Read the model definition and answer for the solid it produces. Units are mm, in the model's axes. A direction names the side the tool comes from. Coordinates: 2 decimals unless noted, no trailing zeros. Order: outer loops, then holes, each group sorted by start corner. A loop starts at its lowest first (then second) coordinate and runs counter-clockwise, first axis right, second up. Notation, with made-up numbers: (85, -10.5) -> (130, -10.5) arc R13 ccw to (130, 10.5) -> close; hole circle Ø1 at (22, 6). An arc over 180 degrees is marked (long way). Use CSV: the item, a comma, the result in double quotes.
```python
from build123d import *

# Parameters (mm, degrees)
BOSS_EXTRUDE1_DEPTH = 50
FILLET1_R           = 4
CUT_EXTRUDE1_DEPTH  = 1.5


with BuildPart() as part:
    # Sketch1 → Boss-Extrude1 (new body)
    with BuildSketch(Plane.XY):
        Polygon((0, 0), (15, 32.788635103), (15, 40), (-3.299023369, 0), align=None)
    extrude(amount=BOSS_EXTRUDE1_DEPTH)

    # Fillet1
    fillet1_edges = [part.edges().sort_by_distance(p)[0] for p in [
        (-1.649511685, 0, 50),
        (-1.649511685, 0, 0),
    ]]
    fillet(fillet1_edges, radius=FILLET1_R)

    # Sketch2 → Cut-Extrude1 (cut)
    with BuildSketch(Plane(origin=(-2.728080099, 1.248030037, 0), x_dir=(0, 0, 1), z_dir=(-0.9093600329934255, 0.4160100123725345, 0))):
        Polygon((20, 12.820411289), (30, 12.820411289), (34.5, 16.820411289), (34.5, 26.820411289), (36.5, 26.820411289), (36.5, 32.820411289), (26, 32.820411289), (26, 26.820411289), (28, 26.820411289), (28, 18.820411289), (22, 18.820411289), (22, 26.820411289), (24, 26.820411289), (24, 32.820411289), (13.5, 32.820411289), (13.5, 26.820411289), (15.5, 26.820411289), (15.5, 16.820411289), align=None)
    extrude(amount=-CUT_EXTRUDE1_DEPTH, mode=Mode.SUBTRACT)


solid = part.part
```
Item 1: A tool of negligible diameter and unlimited length cuts with its end or side. For faces 1 (the flat face through (7, 22, 22)), 2 (the flat face through (3.278, 12.599, 24.93)), 3 (the flat face through (5.774, 18.055, 25.042)), from which of +Z, -Z, +X, -X, +Y, -Y can it reach the whole face along a straight path? Write none if from no direction.
Return value:
face 1,"-X, +Y"
face 2,"+Y"
face 3,"-X"
Item 2: Each of these flat-tipped pins is pushed along its axis until it touches: P1, Ø2, axis at x = 9, z = 21.5, coming from the +Y side; P2, Ø2, axis at y = 30, z = 34, coming from the +X side; P3, Ø3, axis at y = 20, z = 25.5, coming from the +X side; P4, Ø1.9, axis at x = 10, y = 29.5, coming from the -Z side. Where does it stop, or does it pass through?
Return value:
P1,"stops at y = 25.64"
P2,"stops at x = 14.18"
P3,"stops at x = 9.84"
P4,"stops at z = 0"
Item 3: Find section D-D, the plane y = 14. Give the vertices of the cut face in (x, z).
Return value:
outline,"(3.11, 0) -> (6.4, 0) -> (6.4, 50) -> (3.11, 50) -> (3.11, 31.35) -> (4.76, 32.12) -> (4.76, 17.88) -> (3.11, 18.65) -> close"
Item 4: The mould has two halves that part along X. Classify faces 4 (the flat face through (15, 36, 25)), 5 (the cylindrical face through (-0.699, 1.141, 48.797)), 6 (the flat face through (5.98, 20.28, 24.65)), 7 (the flat face through (4.12, 14.44, 17.72)): +X half, -X half, draft (parallel to the pull), parting line (faces both ways), or undercut.
Return value:
face 4,"+X half"
face 5,"draft"
face 6,"-X half"
face 7,"undercut"
Item 5: Straight lines are drawn through the part: line 1 along Y through (x, z) = (11, 17.5) (3 decimals); line 2 along X through (y, z) = (4, 37.5); line 3 along X through (y, z) = (8, 30.5). For each, find the intervals that lie inside material, in ascending order.
Return value:
line 1,"y = 24.045 to 27.651, 31.06 to 31.256"
line 2,"x = -1.47 to 1.83"
line 3,"x = 0.36 to 3.66"
Item 6: Find section C-C, the plane x = 9. Give the vertices of the cut face in (y, z), then the cut area to 3 significant figures.
Return value:
outline,"(19.67, 0) -> (26.88, 0) -> (26.88, 13.5) -> (25.38, 13.5) -> (25.38, 15.5) -> (23.28, 15.5) -> (23.28, 22) -> (25.38, 22) -> (25.38, 24) -> (26.88, 24) -> (26.88, 26) -> (25.38, 26) -> (25.38, 28) -> (23.28, 28) -> (23.28, 34.5) -> (25.38, 34.5) -> (25.38, 36.5) -> (26.88, 36.5) -> (26.88, 50) -> (19.67, 50) -> close"
area,"302 mm^2"
Item 7: Find section A-A, the plane z = 27. Give the vertices of the cut face in (x, y), then the cut area to 3 significant figures.
Return value:
outline,"(-3.3, 0) -> (0, 0) -> (15, 32.79) -> (15, 40) -> (10.93, 31.09) -> (12.29, 30.47) -> (9.79, 25.01) -> (8.43, 25.64) -> (5.1, 18.36) -> (6.47, 17.74) -> (3.97, 12.28) -> (2.61, 12.91) -> close"
area,"102 mm^2"
Item 8: Find section B-B, the plane x = 11.75. Give the vertices of the cut face in (y, z), then the cut area to 3 significant figures.
Return value:
outline,"(25.68, 0) -> (32.9, 0) -> (32.9, 50) -> (25.68, 50) -> close; hole (29.29, 13.5) -> (30.72, 13.5) -> (30.72, 24) -> (29.29, 24) -> close; hole (29.29, 26) -> (30.72, 26) -> (30.72, 36.5) -> (29.29, 36.5) -> close"
area,"331 mm^2"
